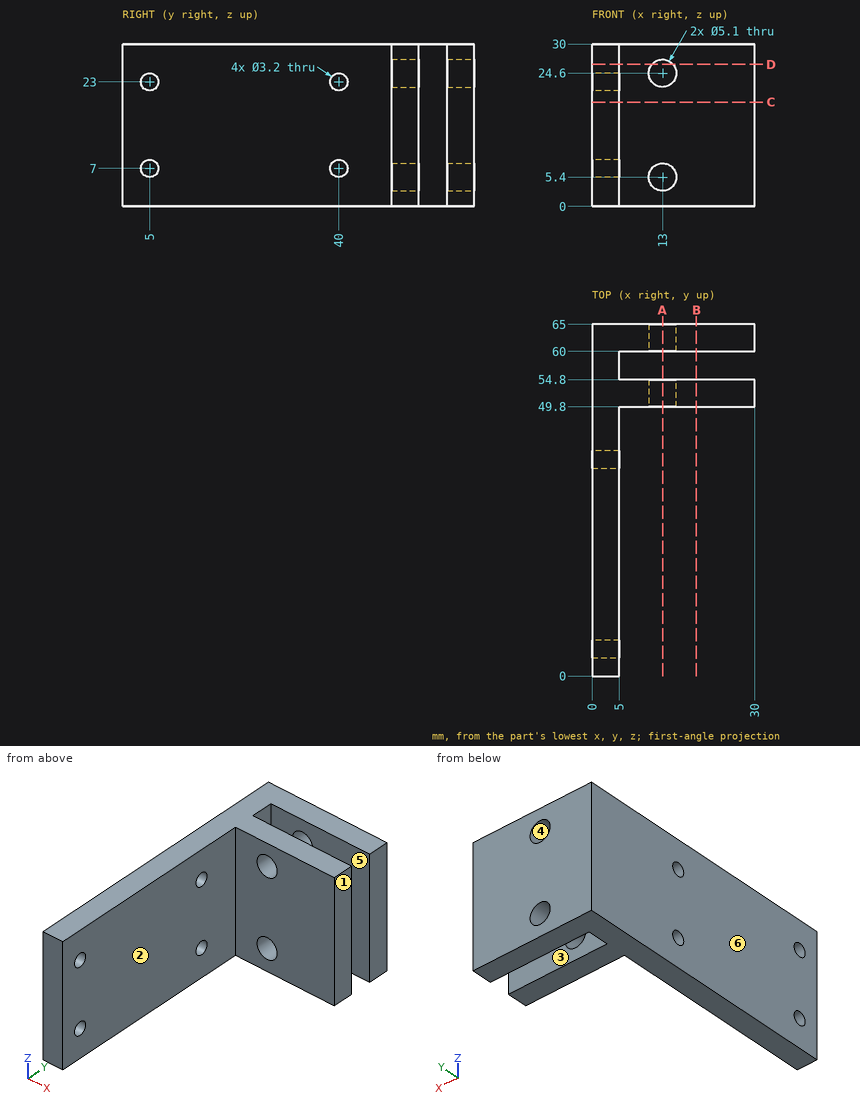
Job drawing, mm, ordinate dimensions from the low corner. One solid piece. A direction names the side the tool comes from. Give positions to 0.01 mm unless a question says otherwise; leave off trailing zeros. Loops run counter-clockwise (first coordinate to the right, second up) from the corner with the lowest first, then second, coordinate; pieces in that order, holes last.
Item 1: Pull direction X, two halves, no side cores. Call the marked faces 4, 5 and 6: released by +X, released by -X, zero draft, split by the parting line, or undercut.
Answers follow:
face 4: undercut
face 5: zero draft
face 6: released by -X
Item 2: Slice it at B-B, the plane x = 19.25. List the corners of the cut face in (y, z), and give its area (3 significant figures).
Answers follow:
outline: (49.8, 0) - (54.8, 0) - (54.8, 30) - (49.8, 30) - close; (60, 0) - (65, 0) - (65, 30) - (60, 30) - close
area: 300 mm2
Item 3: Which spindle directions (+Z, -Z, +X, -X, +Y, -Y) get a long thin tool onto all of the face, cutting with end or side? Do the marked faces 1, 2 and 3. Say none if no direction does.
Answers follow:
face 1: +Z, -Z, +X, +Y, -Y
face 2: +Z, -Z, +X, -Y
face 3: +Z, -Z, +X
Item 4: Drill centre lines: line 1 (Z direction, x = 13, y = 62.85); line 2 (Z direction, x = 2.85, y = 40); line 3 (Y direction, x = 10.5, z = 28.75). Where is each one in solid material? Low to high.
Answers follow:
line 1: z = 0 to 2.85, 7.95 to 22.05, 27.15 to 30
line 2: z = 0 to 5.4, 8.6 to 21.4, 24.6 to 30
line 3: y = 49.8 to 54.8, 60 to 65
Item 5: Flat gauge pins, fed straight in: pin 1 (6 mm diameter, centred on y = 52, z = 23, fed in from -X); pin 2 (4 mm diameter, centred on x = 18.5, z = 14, fed in from -Y); pin 3 (4 mm diameter, centred on x = 13, z = 24.6, fed in from +Y); pin 4 (3.5 mm diameter, centred on y = 5, z = 23, fed in from +X). Where does each tip first touch, or does it go through?
Answers follow:
pin 1: stops at x = 0
pin 2: stops at y = 49.8
pin 3: passes through
pin 4: stops at x = 5
Item 6: Slice it at A-A, the plane x = 13. List the corners of the cut face in (y, z), and give its area (3 significant figures).
Answers follow:
outline: (49.8, 0) - (54.8, 0) - (54.8, 2.85) - (49.8, 2.85) - close; (49.8, 7.95) - (54.8, 7.95) - (54.8, 22.05) - (49.8, 22.05) - close; (49.8, 27.15) - (54.8, 27.15) - (54.8, 30) - (49.8, 30) - close; (60, 0) - (65, 0) - (65, 2.85) - (60, 2.85) - close; (60, 7.95) - (65, 7.95) - (65, 22.05) - (60, 22.05) - close; (60, 27.15) - (65, 27.15) - (65, 30) - (60, 30) - close
area: 198 mm2
Item 7: Slice it at D-D, the plane z = 26.25. List the corners of the cut face in (x, y).
Answers follow:
outline: (0, 0) - (5, 0) - (5, 49.8) - (11.06, 49.8) - (11.06, 54.8) - (5, 54.8) - (5, 60) - (11.06, 60) - (11.06, 65) - (0, 65) - close; (14.94, 49.8) - (30, 49.8) - (30, 54.8) - (14.94, 54.8) - close; (14.94, 60) - (30, 60) - (30, 65) - (14.94, 65) - close
Item 8: Slice it at C-C, the plane z = 19.25. List the corners of the cut face in (x, y), and give its area (3 significant figures).
Answers follow:
outline: (0, 0) - (5, 0) - (5, 49.8) - (30, 49.8) - (30, 54.8) - (5, 54.8) - (5, 60) - (30, 60) - (30, 65) - (0, 65) - close
area: 575 mm2
